Can you work these out from the drawing? Everything is in mm from the part's minimum corner. Round coordinates to 2 decimals unless told otherwise and drop trailing zeros. Write each loop counter-clockwise with the first axis right and the second up, starting at its lowest first coordinate (ties: lowest second). Pieces come first, ordered by that corner, then holes.
Q1. Please list where these lines run through material, in increasing order: line 1 along X through (y, z) = (6.5, 6); line 2 along Y through (x, z) = (6.25, 3); line 3 along Y through (x, z) = (6, 4).
Q2. If we section it at A-A (y = 7): Please give me the cut outline in (x, z), plus the area to 3 significant figures.
Q3. If we section it at B-B (z = 4.75): Please give me the cut outline in (x, y).
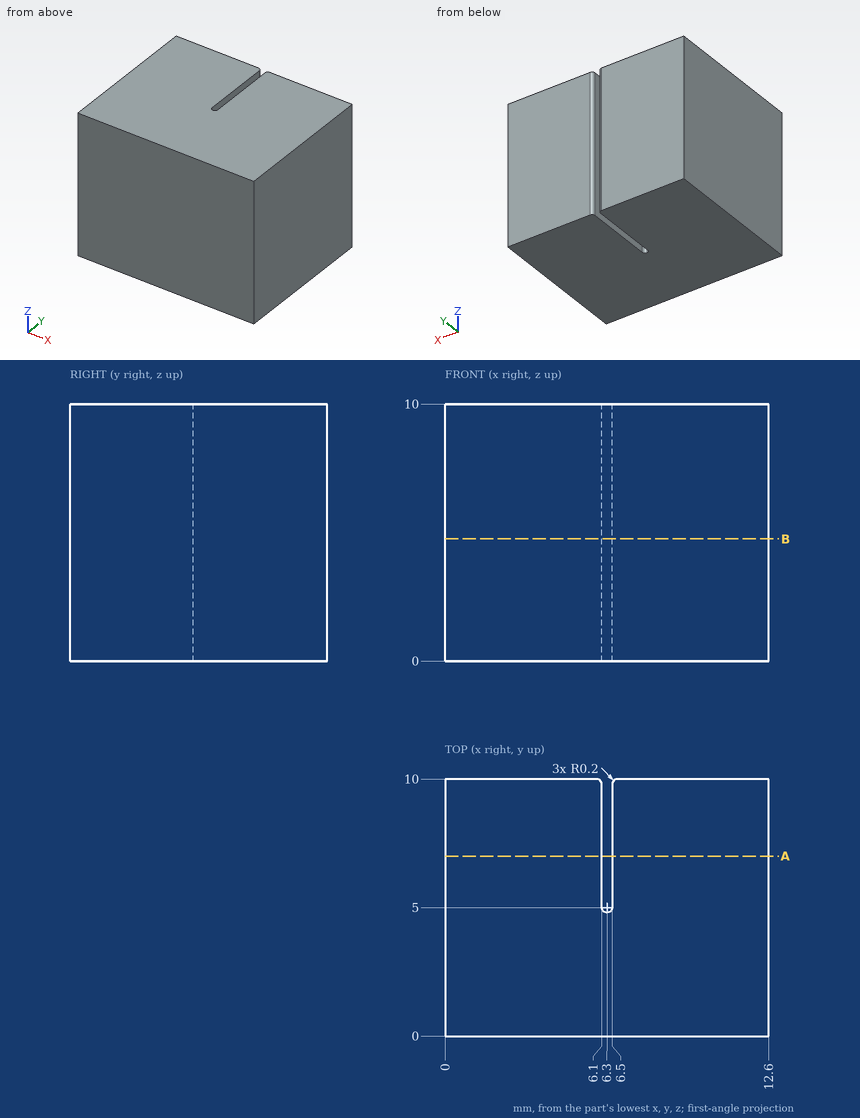
A:
1. line 1: x = 0 to 6.1, 6.5 to 12.6
1. line 2: y = 0 to 4.81
1. line 3: y = 0 to 9.97
2. outline: (0, 0) - (6.1, 0) - (6.1, 10) - (0, 10) - close; (6.5, 0) - (12.6, 0) - (12.6, 10) - (6.5, 10) - close
2. area: 122 mm2
3. outline: (0, 0) - (12.6, 0) - (12.6, 10) - (6.7, 10) arc R0.2 ccw to (6.5, 9.8) - (6.5, 5) arc R0.2 cw to (6.3, 4.8) arc R0.2 cw to (6.1, 5) - (6.1, 9.8) arc R0.2 ccw to (5.9, 10) - (0, 10) - close
